Autodesk Fusion 360 part; units mm, degrees
sketch "Sketch1" plane through (0, 0, 0) normal (0, 0, 1) x (1, 0, 0)
  line L0 (0, 0) -> (19, 0)
  line L1 (0, 0) -> (0, 15)
  line L2 (0, 15) -> (19, 0)
  dimension "d1" = 19
  dimension "d2" = 15
extrude "Extrude1" add sketch "Sketch1" along normal blind 15
sketch "cable_holes" plane through (0, 0, 0) normal (0, -1, 0) x (1, 0, 0)
  line L0 (0, 0) -> (19, 0)
  line L1 (19, 0) -> (19, 15)
  line L2 (19, 15) -> (0, 15)
  line L3 (0, 15) -> (0, 0)
  circle A0 centre (4.2, 10.7) radius 1.7
  circle A1 centre (4.2, 4.3) radius 1.7
  circle A2 centre (12, 7.5) radius 1.7
  line L4 (19, 7.5) -> (0, 7.5) construction
  circle A3 centre (4.2, 10.7) radius 3
  circle A4 centre (4.2, 4.3) radius 3
  circle A5 centre (12, 7.5) radius 3
  dimension "d7" = 3.4
  dimension "d8" = 3.4
  dimension "d9" = 3.4
  dimension "d10" = 4.2
  dimension "d11" = 4.2
  dimension "d12" = 6.4
  dimension "d13" = 12
  dimension "d14" = 4.3
  dimension "d20" = 6
  dimension "d21" = 6
  dimension "d22" = 6
extrude "Extrude2" cut sketch "cable_holes" against normal blind 15 contours A2 | A5
extrude "Extrude4" add sketch "cable_holes" against normal blind 2 contours A5
sketch "Sketch3" plane through (0, 0, 0) normal (-1, 0, 0) x (0, -1, 0)
  line L0 (-15, 0) -> (0, 0)
  line L1 (0, 0) -> (0, 15)
  line L2 (0, 15) -> (-15, 15)
  line L3 (-15, 15) -> (-15, 0)
  circle A0 centre (-7.5, 7.5) radius 1.7
  line L4 (-7.5, 15) -> (-7.5, 0) construction
  line L5 (-15, 7.5) -> (0, 7.5) construction
  circle A1 centre (-7.5, 7.5) radius 3
  dimension "d17" = 3.4
  dimension "d25" = 6
extrude "Extrude3" cut sketch "Sketch3" against normal blind 15 contours A0 | A1
extrude "Extrude5" add sketch "Sketch3" against normal blind 2 contours A1
chamfer "Chamfer1" distance 0.4 angle 45 4 edges at (15, 3.1579, 7.5) (5.7, 10.5, 7.5) (0, 9.085, 8.1147) (10.415, 0, 8.1147)
chamfer "Chamfer2" distance 0.4 angle 45 9 edges at (9.5, 7.5, 15) (0, 7.5, 15) (9.5, 0, 15) (19, 0, 7.5) (0, 15, 7.5) (0, 0, 7.5) (0, 7.5, 0) (9.5, 7.5, 0) (9.5, 0, 0)
equation "inner_hole = 3.4 mm"
equation "outer_hole = 6 mm"
equation "d7 = inner_hole"
equation "d8 = inner_hole"
equation "d9 = inner_hole"
equation "d13 = 4.2 mm + 7.8 mm"
equation "d17 = inner_hole"
equation "d20 = outer_hole"
equation "d21 = outer_hole"
equation "d22 = outer_hole"
equation "d25 = outer_hole"
Can you work these out from the model? Positions are in its coordinate system, mm. A direction names the side the tool comes from. Give positions to 0.01 mm unless a question says otherwise; leave off trailing zeros. Order: outer loops, then holes, each group sorted by start corner. A loop starts at its lowest first (then second) coordinate and runs counter-clockwise, first axis right, second up. Notation, with made-up numbers: (-6.75, 47.5) - (44.25, 47.5) arc R32 cw to (44.25, 81.5) - close; hole circle Ø3 at (15, -15.75). An arc over 180 degrees is marked (long way). Use a Markdown table: item, result. Add a question column.
Q1. If we section it at A-A on z = 2.5: Write out the boundary of the cut face in (x, y), plus the area to 3 significant figures.
Q2. Please list where these lines run through material, in increasing order: line 1 along Z through (x, y) = (4.25, 7.5); line 2 along Z through (x, y) = (1.35, 7.5); line 3 along Y through (x, z) = (4.75, 5.25).
Q3. On a 3-axis mill with a long thin cutter (end or side, diameter ignored), from which of +Z, -Z, +X, -X, +Y, -Y can I reach the whole of each face in a straight line? I mean faces 4 (the flat face through (14, 2, 8)), 5 (the flat face through (9.249, 7.447, 14.797)), 6 (the cylindrical face through (5.29, 4.64, 8.4)). Say none if no direction works.
Q4. If we mould it in two halves opening along Z, with no side actions, what happens to faces 1 (the flat face through (9.67, 7.11, 0.2)), 2 (the flat face through (9, 0, 8)), 3 (the flat face through (2, 6, 6))? For each: released by +Z, released by -Z, zero draft, split by the parting line, or undercut.
Q5. I'm going to push flat-ended pins straight in: pin 1 (6 mm diameter, centred on x = 11, y = 3.5, fed in from -Z); pin 2 (5 mm diameter, centred on x = 7, z = 7, fed in from +Y); pin 3 (5 mm diameter, centred on y = 6.5, z = 8.5, fed in from +X); pin 4 (4 mm diameter, centred on y = 7, z = 1.5, fed in from +X). Where does each tip first touch, or does it pass through?
Answers follow:
| question | item | result |
|---|---|---|
| 1 | outline | (0, 0.4) - (0.4, 0) - (18.6, 0) - (18.69, 0.25) - (0.31, 14.75) - (0, 14.6) - close |
| 1 | area | 142 mm^2 |
| 2 | line 1 | z = 0 to 4.5, 10.5 to 15 |
| 2 | line 2 | z = 0 to 5.8, 9.2 to 15 |
| 2 | line 3 | y = 0 to 5.52, 9.48 to 11.25 |
| 3 | face 4 | +Y |
| 3 | face 5 | +Z, +X, +Y |
| 3 | face 6 | +X |
| 4 | face 1 | released by -Z |
| 4 | face 2 | zero draft |
| 4 | face 3 | undercut |
| 5 | pin 1 | stops at z = 0 |
| 5 | pin 2 | stops at y = 11.45 |
| 5 | pin 3 | stops at x = 12.02 |
| 5 | pin 4 | stops at x = 12.67 |
